Geometry check sheet. Reference: drawing and pictorial views, mm from the part's lowest x, y, z. A direction names the side the tool comes from. Round coordinates to 2 decimals unless told otherwise and drop trailing zeros. Order: outer loops, then holes, each group sorted by start corner. A loop starts at its lowest first (then second) coordinate and runs counter-clockwise, first axis right, second up.
Q1. Cross-section at A-A on z = 23.5. Record the cut outline in (x, y).
Q2. Cross-section at D-D on z = 35. Record the cut outline in (x, y), then the cut area to 3 significant figures.
Q3. Cross-section at C-C on x = 10.5. Record the cut outline in (y, z).
Q4. Depth check by flat-ended pin: P1, Ø4, axis at x = 43.5, y = 6.5, coming from the +Z side; P2, Ø5, axis at x = 16, y = 5.5, coming from the +Z side; P3, Ø7.5, axis at x = 21.5, y = 22, coming from the +Z side. Enter the tip coordinate at first touch or a pass-through.
Q5. Scan lines: probe 1 along X at (y, z) = (26, 22); probe 2 along Z at (x, y) = (24.5, 25.5); probe 3 along Y at (x, z) = (3, 36). Record each from-to range of solid material in increasing order.
Q6. Set-up check for the marked faces 1 and 2: record each of +Z, -Z, +X, -X, +Y, -Y from which the full face is reachable in a straight line by a thin tool's end or side.
Q7. Mould release check, pull along X, two halves, no side actions. Record for the marked faces 3, 4 and 5: +X half, -X half, draft (parallel to the pull), parting line (faces both ways), or undercut.
Q8. Cross-section at B-B on y = 26.5. Record the cut outline in (x, z), then the cut area to 3 significant figures.
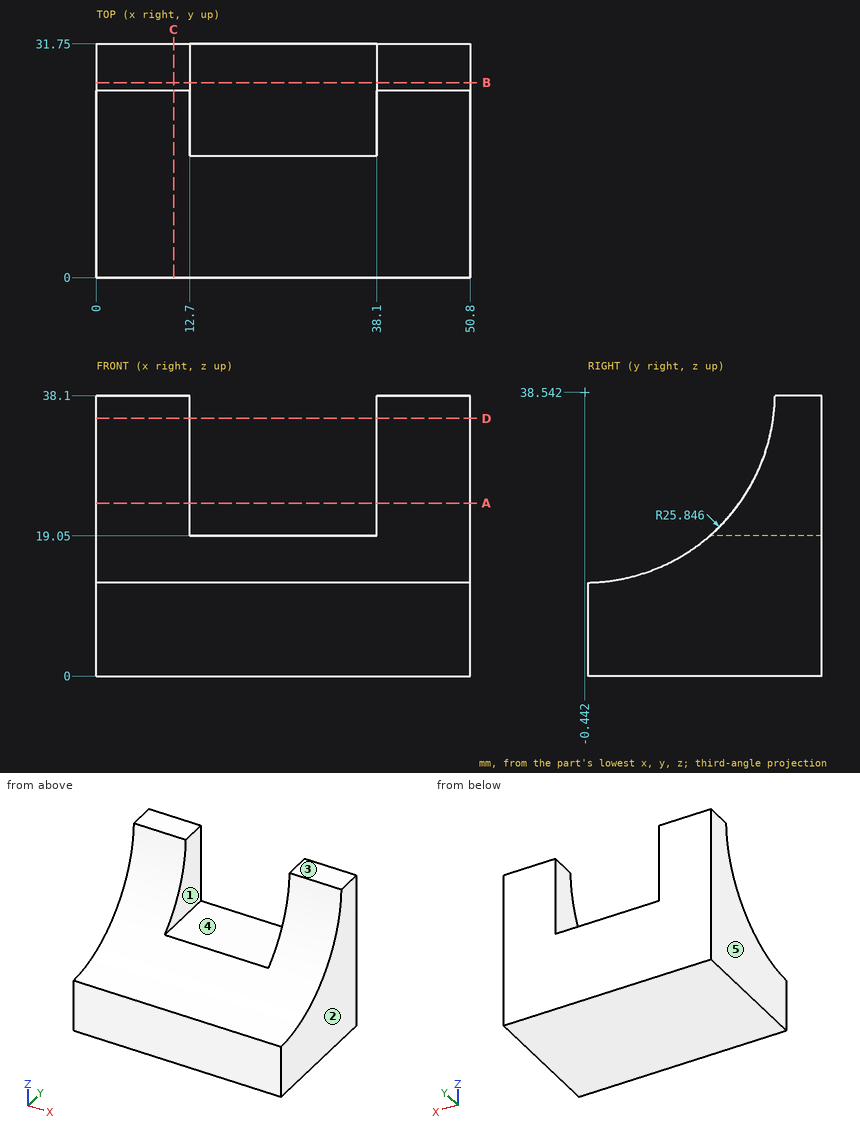
Results found:
1. outline: (0, 20.58) - (12.7, 20.58) - (12.7, 31.75) - (0, 31.75) - close; (38.1, 20.58) - (50.8, 20.58) - (50.8, 31.75) - (38.1, 31.75) - close
2. outline: (0, 25.16) - (12.7, 25.16) - (12.7, 31.75) - (0, 31.75) - close; (38.1, 25.16) - (50.8, 25.16) - (50.8, 31.75) - (38.1, 31.75) - close
2. area: 167 mm2
3. outline: (0, 0) - (31.75, 0) - (31.75, 38.1) - (25.4, 38.1) arc R25.85 cw to (0, 12.7) - close
4. P1: stops at z = 14.29
4. P2: stops at z = 14.11
4. P3: stops at z = 19.05
5. probe 1: x = 0 to 12.7, 38.1 to 50.8
5. probe 2: z = 0 to 19.05
5. probe 3: y = 25.28 to 31.75
6. face 1: +Z, +Y, -Y
6. face 2: +Z, -Z, +X, +Y, -Y
7. face 3: draft
7. face 4: undercut
7. face 5: -X half
8. outline: (0, 0) - (50.8, 0) - (50.8, 38.1) - (38.1, 38.1) - (38.1, 19.05) - (12.7, 19.05) - (12.7, 38.1) - (0, 38.1) - close
8. area: 1,450 mm2
